Geometry: final body of the model. Coordinates: model frame, mm. A direction names the side the tool comes from. Give positions to 0.01 mm unless a question says otherwise; leave off trailing zeros. Write each loop counter-clockwise with the first axis right and the second up, starting at its lowest first coordinate (ties: lowest second). Pieces come first, ordered by that corner, then holes.
Q1. Cut plane B-B on y = 35. Return the cut outline in (x, z).
Q2. Pin query (flat end, axial travel): pin 1 (1 mm diameter, centred on x = 2.5, y = 54, fed in from +Z); pin 2 (5 mm diameter, centred on x = 0, y = 35, fed in from +Z); pin 3 (2.5 mm diameter, centred on x = -63, y = 54.5, fed in from -Z); pin 4 (4.5 mm diameter, centred on x = 0, y = 55, fed in from +Z). Return the tip coordinate at first contact, or that it passes through.
Q3. Line query: L1, parallel to X at y = 55, z = 2.5; L2, parallel to X at y = 20, z = -5; L3, parallel to X at y = 35, z = 3.2. Output: solid intervals per line, ascending.
Q4. Draft query along X for faces 4 (the face through (75.2, 35, -11)), 5 (the face through (1, 43, 5)), 6 (the face through (75.294, 34.51, 2.434)). Return one class per face: pulls with the +X half, pulls with the -X half, needs draft (parallel to the pull), parting line crosses it, or undercut.
Q5. Cut plane D-D on y = 14.5. Return the cut outline in (x, z).
Q6. Reachability of faces 1 (the face through (-63.9, 22.5, 3)), 2 (the face through (71.797, 1.521, -1.141)), 3 (the face through (1, 29, 2.2)) from +Z, -Z, +X, -X, +Y, -Y: full face, straight path, thin tool, end or side. Return the list, or none.
Q7. Cut plane C-C on x = -28.5. Return the cut outline in (y, z).
```python
from build123d import *

# Parameters (mm, degrees)
SKETCH002_R     = 1.5
POCKET_DEPTH    = 23.001
SKETCH003_R     = 4
PAD_DEPTH       = 5.4
SKETCH004_R     = 1
POCKET001_DEPTH = 8.201
SKETCH005_R     = 2.5
POCKET002_DEPTH = 3
CHAMFER_SIZE    = 1
CHAMFER001_SIZE = 1
CHAMFER002_SIZE = 1
CHAMFER003_SIZE = 1
CHAMFER004_SIZE = 1
CHAMFER005_SIZE = 1


with BuildPart() as part:
    # AdditivePipe: sweep along a path in Sketch001
    with BuildLine(Plane.XZ) as additivepipe_path:
        Line((-73, -18), (-73, -4))
        ThreePointArc((-73, -4), (-71.828427, -1.171573), (-69, 0))
        Line((-69, 0), (0, 0))
        Line((0, 0), (69, 0))
        ThreePointArc((69, 0), (71.828427, -1.171573), (73, -4))
        Line((73, -4), (73, -18))
    # Sketch → AdditivePipe (sweep)
    with BuildSketch(Plane.YZ):
        Polygon((0, 5), (70, 5), (70, 0), (67, 0), (67, 2.2), (63.8, 2.2), (63.8, 0), (60.8, 0), (60.8, 2.2), (9.2, 2.2), (9.2, 0), (6.2, 0), (6.2, 2.2), (3, 2.2), (3, 0), (0, 0), align=None)
    sweep(path=additivepipe_path.line)

    # Sketch002 (on Face35 of AdditivePipe) → Pocket (cut, through all)
    with BuildSketch(Plane(origin=(0, 0, 5), x_dir=(0, -1, 0), z_dir=(0, 0, 1))):
        with Locations((-35, -64)):
            Circle(SKETCH002_R)
        with Locations((-35, 64)):
            Circle(SKETCH002_R)
        with Locations((-35, 0)):
            Circle(SKETCH002_R)
    extrude(amount=-POCKET_DEPTH, mode=Mode.SUBTRACT)

    # Sketch003 (on Face43 of Pocket) → Pad (join)
    with BuildSketch(Plane.YX.offset(-2.2)):
        with Locations((20, 64)):
            Circle(SKETCH003_R)
        with Locations((55, 64)):
            Circle(SKETCH003_R)
        with Locations((20, 0)):
            Circle(SKETCH003_R)
        with Locations((55, 0)):
            Circle(SKETCH003_R)
        with Locations((20, -64)):
            Circle(SKETCH003_R)
        with Locations((55, -64)):
            Circle(SKETCH003_R)
    extrude(amount=PAD_DEPTH)

    # Sketch004 (on Face88 of Pad) → Pocket001 (cut, through all)
    with BuildSketch(Plane.YX.offset(3.2)):
        with Locations((20, -64)):
            Circle(SKETCH004_R)
        with Locations((55, -64)):
            Circle(SKETCH004_R)
        with Locations((55, 0)):
            Circle(SKETCH004_R)
        with Locations((20, 0)):
            Circle(SKETCH004_R)
        with Locations((20, 64)):
            Circle(SKETCH004_R)
        with Locations((55, 64)):
            Circle(SKETCH004_R)
    extrude(amount=-POCKET001_DEPTH, mode=Mode.SUBTRACT)

    # Sketch005 (on Face35 of Pocket001) → Pocket002 (cut)
    with BuildSketch(Plane(origin=(0, 0, 5), x_dir=(0, -1, 0), z_dir=(0, 0, 1))):
        with Locations((-55, 64)):
            Circle(SKETCH005_R)
        with Locations((-20, 64)):
            Circle(SKETCH005_R)
        with Locations((-55, 0)):
            Circle(SKETCH005_R)
        with Locations((-20, 0)):
            Circle(SKETCH005_R)
        with Locations((-55, -64)):
            Circle(SKETCH005_R)
        with Locations((-20, -64)):
            Circle(SKETCH005_R)
    extrude(amount=-POCKET002_DEPTH, mode=Mode.SUBTRACT)

    # Chamfer
    chamfer_edges = [part.edges().sort_by_distance(p)[0] for p in [
        (-64, 57.5, 5),
    ]]
    chamfer(chamfer_edges, length=CHAMFER_SIZE)

    # Chamfer001
    chamfer001_edges = [part.edges().sort_by_distance(p)[0] for p in [
        (-2.5, 55, 5),
        (2.5, 55, 5),
    ]]
    chamfer(chamfer001_edges, length=CHAMFER001_SIZE)

    # Chamfer002
    chamfer002_edges = [part.edges().sort_by_distance(p)[0] for p in [
        (64, 57.5, 5),
    ]]
    chamfer(chamfer002_edges, length=CHAMFER002_SIZE)

    # Chamfer003
    chamfer003_edges = [part.edges().sort_by_distance(p)[0] for p in [
        (64, 22.5, 5),
    ]]
    chamfer(chamfer003_edges, length=CHAMFER003_SIZE)

    # Chamfer004
    chamfer004_edges = [part.edges().sort_by_distance(p)[0] for p in [
        (-2.5, 20, 5),
        (2.5, 20, 5),
    ]]
    chamfer(chamfer004_edges, length=CHAMFER004_SIZE)

    # Chamfer005
    chamfer005_edges = [part.edges().sort_by_distance(p)[0] for p in [
        (-64, 22.5, 5),
    ]]
    chamfer(chamfer005_edges, length=CHAMFER005_SIZE)


solid = part.part
```
Data:
1. outline: (-78, -18) - (-75.2, -18) - (-75.2, -4) arc R6.2 cw to (-69, 2.2) - (-65.5, 2.2) - (-65.5, 5) - (-69, 5) arc R9 ccw to (-78, -4) - close; (-62.5, 2.2) - (-1.5, 2.2) - (-1.5, 5) - (-62.5, 5) - close; (1.5, 2.2) - (62.5, 2.2) - (62.5, 5) - (1.5, 5) - close; (65.5, 2.2) - (69, 2.2) arc R6.2 cw to (75.2, -4) - (75.2, -18) - (78, -18) - (78, -4) arc R9 ccw to (69, 5) - (65.5, 5) - close
2. pin 1: stops at z = 4.69
2. pin 2: stops at z = 5
2. pin 3: stops at z = -3.2
2. pin 4: stops at z = 2
3. L1: x = -75.22 to -66.5, -61.5 to -2.5, 2.5 to 61.5, 66.5 to 75.22
3. L2: x = -78 to -75.2, 75.2 to 78
3. L3: x = -74.4 to -65.5, -62.5 to -1.5, 1.5 to 62.5, 65.5 to 74.4
4. face 4: undercut
4. face 5: needs draft
4. face 6: pulls with the +X half
5. outline: (-78, -18) - (-75.2, -18) - (-75.2, -4) arc R6.2 cw to (-69, 2.2) - (69, 2.2) arc R6.2 cw to (75.2, -4) - (75.2, -18) - (78, -18) - (78, -4) arc R9 ccw to (69, 5) - (-69, 5) arc R9 ccw to (-78, -4) - close
6. face 1: +Z
6. face 2: -Z, +Y, -Y
6. face 3: -Z
7. outline: (0, 0) - (3, 0) - (3, 2.2) - (6.2, 2.2) - (6.2, 0) - (9.2, 0) - (9.2, 2.2) - (60.8, 2.2) - (60.8, 0) - (63.8, 0) - (63.8, 2.2) - (67, 2.2) - (67, 0) - (70, 0) - (70, 5) - (0, 5) - close
